from build123d import *

# Parameters (mm, degrees)
BOSS_EXTRUDE1_DEPTH = 32
CHAMFER1_SIZE       = 2
BOSS_EXTRUDE2_DEPTH = 6
SKETCH11_R          = 11
SKETCH11_R_2        = 7
BOSS_EXTRUDE3_DEPTH = 10
CUT_EXTRUDE1_START  = -6
SKETCH14_R          = 7
CUT_EXTRUDE1_DEPTH  = 6


with BuildPart() as part:
    # Sketch1 → Boss-Extrude1 (new body)
    with BuildSketch(Plane.XY):
        Polygon((0, -1.708319116), (0, 32.291680884), (-23, 32.291680884), (-23, 40.291680884), (31, 40.291680884), (31, 32.291680884), (8, 32.291680884), (8, -1.708319116), align=None)
    extrude(amount=-BOSS_EXTRUDE1_DEPTH)

    # Chamfer1
    chamfer1_edges = [part.edges().sort_by_distance(p)[0] for p in [
        (-23, 36.291680884, 0),
        (31, 36.291680884, 0),
    ]]
    chamfer(chamfer1_edges, length=CHAMFER1_SIZE)

    # Sketch5 → Boss-Extrude2 (add)
    with BuildSketch(Plane(origin=(0, 0, -32), x_dir=(-1, 0, 0), z_dir=(0, 0, -1))):
        Polygon((23, 40.291680884), (-31, 40.291680884), (-21, 78.291680884), (13, 78.291680884), align=None)
    extrude(amount=-BOSS_EXTRUDE2_DEPTH)

    # Sketch11 → Boss-Extrude3 (add)
    with BuildSketch(Plane.XY.offset(-26)):
        with Locations((4, 59.291680884)):
            Circle(SKETCH11_R)
        with Locations((4, 59.291680884)):
            Circle(SKETCH11_R_2, mode=Mode.SUBTRACT)
    extrude(amount=BOSS_EXTRUDE3_DEPTH)

    # Sketch14 → Cut-Extrude1 (cut)
    with BuildSketch(Plane.XY.offset(-26).offset(CUT_EXTRUDE1_START)):
        with Locations((4, 59.291680884)):
            Circle(SKETCH14_R)
    extrude(amount=CUT_EXTRUDE1_DEPTH, mode=Mode.SUBTRACT)


solid = part.part
Input: part model. Units: mm. Frame: model coordinates. A direction names the side the tool comes from. Round coordinates to 2 decimals unless told otherwise and drop trailing zeros. Loops run counter-clockwise (first coordinate to the right, second up) from the corner with the lowest first, then second, coordinate; pieces in that order, holes last. Notation, with made-up numbers: M 80.25,56.5 L 101.25,56.5 A14 cw 101.25,78.5 Z; hole C 16,0.5 d10. An arc over 180 degrees is marked long. Answer as CSV lines item,"result". Start each with the question number.
(1) First-contact query: pin 1 (5 mm diameter, centred on x = -8.5, z = -18.5, fed in from -Y); pin 2 (19 mm diameter, centred on x = -9, y = 51.5, fed in from +Z); pin 3 (8 mm diameter, centred on x = 7, z = -9, fed in from +Y). Flat tips, straight axial feed; report the tip coordinate or a pass-through.
(2) Section D-D, the plane y = 69. Output: boundary loops of the cut face in (x, z).
(3) Reachability of faces 4 (the flat face through (8, 16, -16)), 5 (the cylindrical face through (9.91, 68.57, -21.07)), 6 (the flat face through (11.2, 59.4, -16)) from +Z, -Z, +X, -X, +Y, -Y: full face, straight path, thin tool, end or side. Return the list, or none.
(4) Section C-C, the plane x = -4. Output: boundary loops of the cut face in (y, z), plus the area to 3 significant figures.
(5) Section A-A, the plane x = 4. Output: boundary loops of the cut face in (y, z), plus the area to 3 significant figures.
(6) Section B-B, the plane z = -5. Output: boundary loops of the cut face in (x, y), plus the area to 3 significant figures.
(7) Draft query along X for faces 1 (the cylindrical face through (3.089, 66.232, -24.112)), 2 (the flat face through (20, 32.292, -16)), 3 (the flat face through (0, 15, -16)). Return one class per face: released by +X, released by -X, zero draft, split by the parting line, or undercut.
(8) Line query: line 1 (Y direction, x = 4, z = -23.75); line 2 (Y direction, x = 5, z = -25); line 3 (Y direction, x = 28, z = -6). Output: solid intervals per line, ascending. Write a range as [from, to].
Values found:
1,pin 1,"stops at y = 32.29"
1,pin 2,"stops at z = -16"
1,pin 3,"stops at y = 40.29"
2,outline,"M -15.45,-32 L 23.45,-32 L 23.45,-26 L 9.17,-26 L 9.17,-16 L -1.17,-16 L -1.17,-26 L -15.45,-26 Z"
3,face 4,"+Z, -Z, +X, -Y"
3,face 5,"+Z"
3,face 6,"+Z, +X, -X, +Y"
4,outline,"M 32.29,-32 L 78.29,-32 L 78.29,-26 L 66.84,-26 L 66.84,-16 L 51.74,-16 L 51.74,-26 L 40.29,-26 L 40.29,0 L 32.29,0 Z"
4,area,"635 mm²"
5,outline,"M -1.71,-32 L 52.29,-32 L 52.29,-16 L 48.29,-16 L 48.29,-26 L 40.29,-26 L 40.29,0 L -1.71,0 Z; M 66.29,-32 L 78.29,-32 L 78.29,-26 L 70.29,-26 L 70.29,-16 L 66.29,-16 Z"
5,area,"1,570 mm²"
6,outline,"M -23,32.29 L 0,32.29 L 0,-1.71 L 8,-1.71 L 8,32.29 L 31,32.29 L 31,40.29 L -23,40.29 Z"
6,area,"704 mm²"
7,face 1,"undercut"
7,face 2,"zero draft"
7,face 3,"released by -X"
8,line 1,"y = [-1.71, 40.29], [48.29, 52.29], [66.29, 70.29]"
8,line 2,"y = [-1.71, 40.29], [48.34, 52.36], [66.22, 70.25]"
8,line 3,"y = [32.29, 40.29]"
